```python
from build123d import *

# Parameters (mm, degrees)
SKETCH1_R           = 11.7
BOSS_EXTRUDE1_DEPTH = 24.5
SKETCH2_R           = 10.85
CUT_EXTRUDE1_DEPTH  = 0.3
SKETCH3_R           = 8.4
BOSS_EXTRUDE2_DEPTH = 0.3
SKETCH6_R           = 0.75
BOSS_EXTRUDE3_DEPTH = 6
FILLET12_R          = 0.7


with BuildPart() as part:
    # Sketch1 → Boss-Extrude1 (new body)
    with BuildSketch(Plane(origin=(0, 0, 0), x_dir=(1, 0, 0), z_dir=(0, 1, 0))):
        with Locations(Location((0, 0, 0), (0, 0, 270))):
            Circle(SKETCH1_R)
    extrude(amount=BOSS_EXTRUDE1_DEPTH)

    # Sketch2 → Cut-Extrude1 (cut)
    with BuildSketch(Plane(origin=(0, 24.5, 0), x_dir=(1, 0, 0), z_dir=(0, 1, 0))):
        with Locations(Location((0, 0, 0), (0, 0, 270))):
            Circle(SKETCH2_R)
    extrude(amount=-CUT_EXTRUDE1_DEPTH, mode=Mode.SUBTRACT)

    # Sketch3 → Boss-Extrude2 (add)
    with BuildSketch(Plane(origin=(0, 24.2, 0), x_dir=(1, 0, 0), z_dir=(0, 1, 0))):
        with Locations(Location((0, 0, 0), (0, 0, 270))):
            Circle(SKETCH3_R)
    extrude(amount=BOSS_EXTRUDE2_DEPTH)

    # Sketch6 → Boss-Extrude3 (add)
    with BuildSketch(Plane.XZ):
        with Locations(Location((7.5, 0, 0), (0, 0, 90))):
            Circle(SKETCH6_R)
        with Locations(Location((3.75, 6.495190528, 0), (0, 0, 90))):
            Circle(SKETCH6_R)
        with Locations(Location((-3.75, 6.495190528, 0), (0, 0, 90))):
            Circle(SKETCH6_R)
        with Locations(Location((3.75, -6.495190528, 0), (0, 0, 90))):
            Circle(SKETCH6_R)
        with Locations(Location((-3.75, -6.495190528, 0), (0, 0, 90))):
            Circle(SKETCH6_R)
    extrude(amount=BOSS_EXTRUDE3_DEPTH)

    # Fillet12
    fillet12_edges = [part.edges().sort_by_distance(p)[0] for p in [
        (7.5, -6, -0.75),
        (3.75, -6, 5.745190528),
        (-3.75, -6, 5.745190528),
        (3.75, -6, -7.245190528),
        (-3.75, -6, -7.245190528),
    ]]
    fillet(fillet12_edges, radius=FILLET12_R)


solid = part.part
```
Model file for the job. Use its own axes, mm. A direction names the side the tool comes from. Coordinates: 2 decimals unless noted, no trailing zeros. Write each loop counter-clockwise with the first axis right and the second up, starting at its lowest first coordinate (ties: lowest second). Pieces come first, ordered by that corner, then holes. Notation, with made-up numbers: (-37, 42.25) - (0, 42.25) arc R14 ccw to (0, 55.25) - close; hole circle Ø7 at (45.25, -33). An arc over 180 degrees is marked (long way). One line per question, with ' | ' between items. Start each with the question number.
Q1. Cut at C-C, the plane y = 8. List the corners of the cut face in (x, z).
Q2. Drill centre lines: line 1 (X direction, y = 24.45, z = 0); line 2 (Y direction, x = -0.5, z = -9); line 3 (Z direction, x = -0.25, y = 1.5). Where is each one in solid material? Low to high. Write a range as [from, to].
Q3. Pin check, flat tips, straight feed: pin 1 (10 mm diameter, centred on x = -7.5, y = 10, fed in from +Z); pin 2 (1 mm diameter, centred on y = 2, z = 2.5, fed in from -X); pin 3 (4 mm diameter, centred on x = 6.5, y = 5.5, fed in from -Z). Stop position of each tip, or through.
Q4. Cut at A-A, the plane x = 0. List the corners of the cut face in (y, z).
Q5. 3-axis set-ups, long thin cutter, end or side, ignore diameter. For faces 1 (the face through (9.15, 24.35, 5.83)), 2 (the face through (-10.38, 12.08, 5.4)), 3 (the face through (7.275, -2.613, 0.715)): which of +Z, -Z, +X, -X, +Y, -Y reach the whole face in a straight line?
Q6. Cut at D-D, the plane z = 9.25. List the corners of the cut face in (x, y), then the cut area to 3 significant figures.
Q7. Cut at B-B, the plane z = -2.75. List the corners of the cut face in (x, y), then the cut area to 3 significant figures.
Answer below:
1) outline: circle Ø23.4 at (0, 0)
2) line 1: [-11.7, -10.85], [-8.4, 8.4], [10.85, 11.7] | line 2: [0, 24.2] | line 3: [-11.7, 11.7]
3) pin 1: z = 11.43 | pin 2: x = -11.53 | pin 3: z = -10.8
4) outline: (0, -11.7) - (24.5, -11.7) - (24.5, -10.85) - (24.2, -10.85) - (24.2, -8.4) - (24.5, -8.4) - (24.5, 8.4) - (24.2, 8.4) - (24.2, 10.85) - (24.5, 10.85) - (24.5, 11.7) - (0, 11.7) - close
5) face 1: +Y | face 2: +Y, -Y | face 3: -Y
6) outline: (-7.16, 0) - (7.16, 0) - (7.16, 24.5) - (5.67, 24.5) - (5.67, 24.2) - (-5.67, 24.2) - (-5.67, 24.5) - (-7.16, 24.5) - close | area: 348 mm^2
7) outline: (-11.37, 0) - (11.37, 0) - (11.37, 24.5) - (10.5, 24.5) - (10.5, 24.2) - (7.94, 24.2) - (7.94, 24.5) - (-7.94, 24.5) - (-7.94, 24.2) - (-10.5, 24.2) - (-10.5, 24.5) - (-11.37, 24.5) - close | area: 556 mm^2
